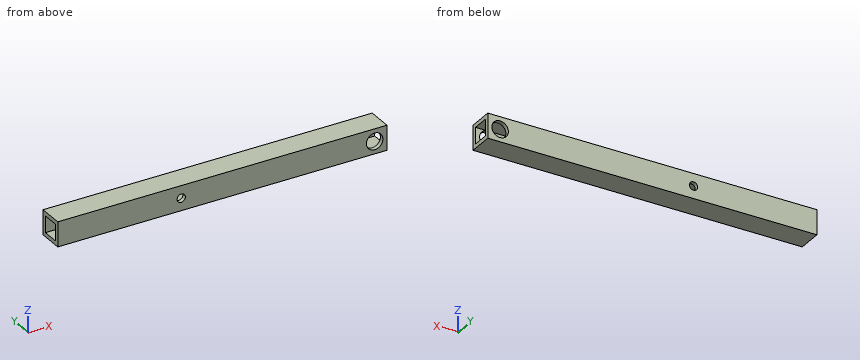
from build123d import *

# Parameters (mm, degrees)
SKETCH1_W           = 15
SKETCH1_H           = 15
SKETCH1_W_2         = 10
SKETCH1_H_2         = 10
BOSS_EXTRUDE1_DEPTH = 200
SKETCH2_R           = 5
CUT_EXTRUDE1_DEPTH  = 16
SKETCH3_R           = 2.5
CUT_EXTRUDE2_DEPTH  = 100


with BuildPart() as part:
    # Sketch1 → Boss-Extrude1 (new body)
    with BuildSketch(Plane(origin=(0, 0, 0), x_dir=(0, 0, -1), z_dir=(1, 0, 0))):
        Rectangle(SKETCH1_W, SKETCH1_H)
        Rectangle(SKETCH1_W_2, SKETCH1_H_2, mode=Mode.SUBTRACT)
    extrude(amount=BOSS_EXTRUDE1_DEPTH)

    # Sketch2 → Cut-Extrude1 (cut, through all)
    with BuildSketch(Plane(origin=(0, 7.5, 0), x_dir=(1, 0, 0), z_dir=(0, 1, 0))):
        with Locations((192.5, 0)):
            Circle(SKETCH2_R)
    extrude(amount=-CUT_EXTRUDE1_DEPTH, mode=Mode.SUBTRACT)

    # Sketch3 → Cut-Extrude2 (cut)
    with BuildSketch(Plane(origin=(0, 7.5, 0), x_dir=(1, 0, 0), z_dir=(0, 1, 0))):
        with Locations((75, 0)):
            Circle(SKETCH3_R)
    extrude(amount=-CUT_EXTRUDE2_DEPTH, mode=Mode.SUBTRACT)


solid = part.part
Geometry check sheet. Reference: the model listing, model coordinates, mm. Coordinates: 2 decimals unless noted, no trailing zeros. Order: outer loops, then holes, each group sorted by start corner. A loop starts at its lowest first (then second) coordinate and runs counter-clockwise, first axis right, second up. Notation, with made-up numbers: M -17.75,84.25 L 17.25,84.25 A27 ccw 17.25,104.25 Z; hole C -11,24 d3. An arc over 180 degrees is marked long. Use CSV: the item, a comma, the result in double quotes.
Item 1: Cross-section at B-B on z = 0. Record the cut outline in (x, y), then the cut area to 3 significant figures.
Returned:
outline,"M 0,-7.5 L 72.5,-7.5 L 72.5,-5 L 0,-5 Z; M 0,5 L 72.5,5 L 72.5,7.5 L 0,7.5 Z; M 77.5,-7.5 L 187.5,-7.5 L 187.5,-5 L 77.5,-5 Z; M 77.5,5 L 187.5,5 L 187.5,7.5 L 77.5,7.5 Z; M 197.5,-7.5 L 200,-7.5 L 200,-5 L 197.5,-5 Z; M 197.5,5 L 200,5 L 200,7.5 L 197.5,7.5 Z"
area,"925 mm2"
Item 2: Cross-section at A-A on x = 98. Record the cut outline in (y, z).
Returned:
outline,"M -7.5,-7.5 L 7.5,-7.5 L 7.5,7.5 L -7.5,7.5 Z; hole M -5,-5 L 5,-5 L 5,5 L -5,5 Z"
Item 3: Thickness scan on line 1 along X through (y, z) = (6.1, 0); line 2 along Y through (x, z) = (108, -4.25). Record the ranges inside material, lowest first.
Returned:
line 1,"x = 0 to 72.5, 77.5 to 187.5, 197.5 to 200"
line 2,"y = -7.5 to -5, 5 to 7.5"
Item 4: Cross-section at C-C on y = -0.75. Record the cut outline in (x, z), then the cut area to 3 significant figures.
Returned:
outline,"M 0,-7.5 L 200,-7.5 L 200,-5 L 0,-5 Z; M 0,5 L 200,5 L 200,7.5 L 0,7.5 Z"
area,"1,000 mm2"
Item 5: Cross-section at D-D on x = 75. Record the cut outline in (y, z).
Returned:
outline,"M -7.5,-7.5 L 7.5,-7.5 L 7.5,-2.5 L 5,-2.5 L 5,-5 L -5,-5 L -5,-2.5 L -7.5,-2.5 Z; M -7.5,2.5 L -5,2.5 L -5,5 L 5,5 L 5,2.5 L 7.5,2.5 L 7.5,7.5 L -7.5,7.5 Z"
